from build123d import *

# Parameters (mm, degrees)
SKETCH2_R           = 11
SKETCH2_R_2         = 5
SKETCH2_R_3         = 1.5
SKETCH2_R_4         = 4
SKETCH2_R_5         = 1.75
SKETCH2_RX          = 4
SKETCH2_RY          = 4
SKETCH2_RX_2        = 1.5
SKETCH2_RY_2        = 1.499925
SKETCH2_RX_3        = 3.75
SKETCH2_RY_3        = 3.7498125
BOSS_EXTRUDE1_DEPTH = 2


with BuildPart() as part:
    # Sketch2 → Boss-Extrude1 (new body)
    with BuildSketch(Plane(origin=(0, 0, 0), x_dir=(1, 0, 0), z_dir=(0, 1, 0))):
        with BuildLine():
            Line((-106.00499968, 144.943614194), (182.962816245, 145.197156615))
            add(Edge.make_bspline(
                [(214.069631291, 100.332253712), (230.927799732, 145.239327045), (182.962816245, 145.197156615)],
                knots=[4.353250182, 4.353250182, 4.353250182, 6.284064455, 6.284064455, 6.284064455], degree=2, weights=[1, 0.569082143, 1]))
            Line((214.069631291, 100.332253712), (171.90071668, -12.000000001))
            add(Edge.make_bspline(
                [(160.992350179, -19), (168.692373591, -19.000128232), (171.90071668, -12.000000001)],
                knots=[3.141576001, 3.141576001, 3.141576001, 4.282613549, 4.282613549, 4.282613549], degree=2, weights=[1, 0.841620915, 1]))
            Line((160.992350179, -19), (-18.998606102, -18.99996049))
            add(Edge.make_bspline(
                [(-29.699861268, -12.428586042), (-26.366669696, -18.999958873), (-18.998606102, -18.99996049)],
                knots=[5.181825727, 5.181825727, 5.181825727, 6.283185508, 6.283185508, 6.283185508], degree=2, weights=[1, 0.852168955, 1]))
            Line((-29.699861268, -12.428586042), (-116.08526313, 126.611232779))
            add(Edge.make_bspline(
                [(-106.00499968, 144.943614194), (-127.678824036, 144.924558741), (-116.08526313, 126.611232779)],
                knots=[0.000879148, 0.000879148, 0.000879148, 2.135198153, 2.135198153, 2.135198153], degree=2, weights=[1, 0.482613975, 1]))
        make_face()
        with Locations((182.992000002, 111.999999999)):
            Circle(SKETCH2_R, mode=Mode.SUBTRACT)
        with Locations((-18.9988, 64)):
            Circle(SKETCH2_R_2, mode=Mode.SUBTRACT)
        with Locations((70.99645, 64)):
            Circle(SKETCH2_R_2, mode=Mode.SUBTRACT)
        with Locations((150.9927, 64)):
            Circle(SKETCH2_R_2, mode=Mode.SUBTRACT)
        with Locations((-78.996040132, 136.5)):
            Circle(SKETCH2_R_3, mode=Mode.SUBTRACT)
        with Locations((20.99895, 136.5)):
            Circle(SKETCH2_R_3, mode=Mode.SUBTRACT)
        with Locations((120.99395, 136.5)):
            Circle(SKETCH2_R_3, mode=Mode.SUBTRACT)
        with Locations((180.99095, 136.5)):
            Circle(SKETCH2_R_3, mode=Mode.SUBTRACT)
        with Locations((170.332531489, 6.118627774)):
            Circle(SKETCH2_R_3, mode=Mode.SUBTRACT)
        with Locations((177.330672341, 24.854456596)):
            Circle(SKETCH2_R_3, mode=Mode.SUBTRACT)
        with Locations((184.328557385, 43.589600555)):
            Circle(SKETCH2_R_3, mode=Mode.SUBTRACT)
        with Locations((191.32646769, 62.324812144)):
            Circle(SKETCH2_R_3, mode=Mode.SUBTRACT)
        with Locations((198.324441471, 81.060193672)):
            Circle(SKETCH2_R_3, mode=Mode.SUBTRACT)
        with Locations((-38.361920415, 16.671266638)):
            Circle(SKETCH2_R_3, mode=Mode.SUBTRACT)
        with Locations((-48.916261932, 33.658786529)):
            Circle(SKETCH2_R_3, mode=Mode.SUBTRACT)
        with Locations((-59.470762984, 50.646563195)):
            Circle(SKETCH2_R_3, mode=Mode.SUBTRACT)
        with Locations((-70.02547384, 67.634677545)):
            Circle(SKETCH2_R_3, mode=Mode.SUBTRACT)
        with Locations((-80.580283096, 84.622950275)):
            Circle(SKETCH2_R_3, mode=Mode.SUBTRACT)
        with Locations((70.99665, -7)):
            Circle(SKETCH2_R_4, mode=Mode.SUBTRACT)
        with Locations((120.99395, 0.5)):
            Circle(SKETCH2_R_5, mode=Mode.SUBTRACT)
        with Locations((20.99895, 0.5)):
            Circle(SKETCH2_R_5, mode=Mode.SUBTRACT)
        with Locations(Location((-105.9945, 133), (0, 0, 180))):
            Ellipse(SKETCH2_RX, SKETCH2_RY, mode=Mode.SUBTRACT)
        with Locations(Location((160.99255, -7), (0, 0, 90))):
            Ellipse(SKETCH2_RX, SKETCH2_RY, mode=Mode.SUBTRACT)
        with Locations(Location((182.99085, 126), (0, 0, 90))):
            Ellipse(SKETCH2_RX_2, SKETCH2_RY_2, mode=Mode.SUBTRACT)
        with Locations(Location((196.99015, 112), (0, 0, 90))):
            Ellipse(SKETCH2_RX_2, SKETCH2_RY_2, mode=Mode.SUBTRACT)
        with Locations(Location((168.99155, 112), (0, 0, 90))):
            Ellipse(SKETCH2_RX_2, SKETCH2_RY_2, mode=Mode.SUBTRACT)
        with Locations(Location((182.99085, 98), (0, 0, 90))):
            Ellipse(SKETCH2_RX_2, SKETCH2_RY_2, mode=Mode.SUBTRACT)
        with Locations(Location((120.99395, 64), (0, 0, 90))):
            Ellipse(SKETCH2_RX_2, SKETCH2_RY_2, mode=Mode.SUBTRACT)
        with Locations(Location((20.99895, 64), (0, 0, 90))):
            Ellipse(SKETCH2_RX_2, SKETCH2_RY_2, mode=Mode.SUBTRACT)
        with Locations(Location((-58.99705, 64), (0, 0, 90))):
            Ellipse(SKETCH2_RX_2, SKETCH2_RY_2, mode=Mode.SUBTRACT)
        with Locations(Location((180.99095, 64), (0, 0, 90))):
            Ellipse(SKETCH2_RX_2, SKETCH2_RY_2, mode=Mode.SUBTRACT)
        with Locations(Location((60.99695, 96.5), (0, 0, 90))):
            Ellipse(SKETCH2_RX_2, SKETCH2_RY_2, mode=Mode.SUBTRACT)
        with Locations(Location((140.99295, 96.5), (0, 0, 90))):
            Ellipse(SKETCH2_RX_2, SKETCH2_RY_2, mode=Mode.SUBTRACT)
        with Locations(Location((160.99195, 31.499978192), (0, 0, 90))):
            Ellipse(SKETCH2_RX_2, SKETCH2_RY_2, mode=Mode.SUBTRACT)
        with Locations(Location((80.99595, 31.499985778), (0, 0, 90))):
            Ellipse(SKETCH2_RX_2, SKETCH2_RY_2, mode=Mode.SUBTRACT)
        with Locations(Location((-18.99905, 96.5), (0, 0, 90))):
            Ellipse(SKETCH2_RX_2, SKETCH2_RY_2, mode=Mode.SUBTRACT)
        with Locations(Location((-38.99805, 31.499994311), (0, 0, 90))):
            Ellipse(SKETCH2_RX_2, SKETCH2_RY_2, mode=Mode.SUBTRACT)
        with Locations(Location((-101.689209002, 118.598380963), (0, 0, 90))):
            Ellipse(SKETCH2_RX_2, SKETCH2_RY_2, mode=Mode.SUBTRACT)
        with Locations(Location((-91.134705429, 101.610600241), (0, 0, 90))):
            Ellipse(SKETCH2_RX_2, SKETCH2_RY_2, mode=Mode.SUBTRACT)
        with Locations(Location((205.322481122, 99.795751553), (0, 0, 90))):
            Ellipse(SKETCH2_RX_2, SKETCH2_RY_2, mode=Mode.SUBTRACT)
        with Locations(Location((20.99895, 96.5), (0, 0, 90))):
            Ellipse(SKETCH2_RX_2, SKETCH2_RY_2, mode=Mode.SUBTRACT)
        with Locations(Location((100.99495, 96.5), (0, 0, 90))):
            Ellipse(SKETCH2_RX_2, SKETCH2_RY_2, mode=Mode.SUBTRACT)
        with Locations(Location((-58.99705, 96.5), (0, 0, 90))):
            Ellipse(SKETCH2_RX_2, SKETCH2_RY_2, mode=Mode.SUBTRACT)
        with Locations(Location((0.99995, 31.499992415), (0, 0, 90))):
            Ellipse(SKETCH2_RX_2, SKETCH2_RY_2, mode=Mode.SUBTRACT)
        with Locations(Location((40.99795, 31.499988622), (0, 0, 90))):
            Ellipse(SKETCH2_RX_2, SKETCH2_RY_2, mode=Mode.SUBTRACT)
        with Locations(Location((120.99395, 31.499981037), (0, 0, 90))):
            Ellipse(SKETCH2_RX_2, SKETCH2_RY_2, mode=Mode.SUBTRACT)
        with Locations(Location((-66.99665, 112), (0, 0, 90))):
            Ellipse(SKETCH2_RX_3, SKETCH2_RY_3, mode=Mode.SUBTRACT)
        with Locations(Location((57.9973, 112), (0, 0, 180))):
            Ellipse(SKETCH2_RX, SKETCH2_RY, mode=Mode.SUBTRACT)
        with Locations(Location((-5.9995, 133), (0, 0, 90))):
            Ellipse(SKETCH2_RX, SKETCH2_RY, mode=Mode.SUBTRACT)
        with Locations(Location((93.995420809, 133), (0, 0, 180))):
            Ellipse(SKETCH2_RX, SKETCH2_RY, mode=Mode.SUBTRACT)
        with BuildLine():
            Line((-18.998603467, -3), (1.00035, -3))
            add(Edge.make_bspline(
                [(1.00035, -11), (5.00035, -11), (5.00035, -7), (5.00035, -3), (1.00035, -3)],
                knots=[3.141592654, 3.141592654, 3.141592654, 4.71238898, 4.71238898, 6.283185307, 6.283185307, 6.283185307], degree=2, weights=[1, 0.707106781, 1, 0.707106781, 1]))
            Line((1.00035, -11), (-18.998603467, -11))
            add(Edge.make_bspline(
                [(-18.998603467, -3), (-22.998556935, -3), (-22.998556935, -7), (-22.998556935, -11), (-18.998603467, -11)],
                knots=[3.141592654, 3.141592654, 3.141592654, 4.71238898, 4.71238898, 6.283185307, 6.283185307, 6.283185307], degree=2, weights=[1, 0.707106781, 1, 0.707106781, 1]))
        make_face(mode=Mode.SUBTRACT)
    extrude(amount=BOSS_EXTRUDE1_DEPTH)


solid = part.part
Check sheet for the modelled part. Datum: model origin and axes. Units: mm. Round coordinates to 2 decimals unless told otherwise and drop trailing zeros. Loops run counter-clockwise (first coordinate to the right, second up) from the corner with the lowest first, then second, coordinate; pieces in that order, holes last. Notation, with made-up numbers: (3.25, 19.25) - (9.25, 19.25) arc R22 ccw to (9.25, 48.25) - close; hole circle Ø2 at (59.25, 69.25). An arc over 180 degrees is marked (long way). Answer as CSV lines item,"result". Start each with the question number.
Item 1: Section check C-C (x = -33). Record the boundary of the cut face in (y, z).
Item 2: Release check for a two-part mould opening along Z. For faces 1 (the flat face through (54, 0, -64)), 2 (the cylindrical face through (74.692, 0.986, 8.532)), 3 (the flat face through (-72.29, 0.99, -56.12)) record: +Z half, -Z half, draft (parallel to the pull), parting line (faces both ways), or undercut.
Item 3: Section check A-A (z = 7). Count the separate pieces of the cut face and the enclosed holes in it, and give its area (3 significant figures).
Item 4: Depth check by flat-ended pin: P1, Ø8, axis at x = 150.99, z = -64, coming from the +Y side; P2, Ø1, axis at x = -9, y = 1, coming from the -Z side. Enter the tip coordinate at first touch or a pass-through.
Item 5: Scan lines: line 1 (Z direction, x = 161, y = 1.35); line 2 (Z direction, x = -5.5, y = 0.4); line 3 (Z direction, x = 22, y = 1.95). Record each from-to range of solid material in increasing order. Write a range as [from, to].
Report:
1,outline,"(0, -145.01) - (2, -145.01) - (2, 7.12) - (0, 7.12) - close"
2,face 1,"draft"
2,face 2,"undercut"
2,face 3,"+Z half"
3,separate pieces,"4"
3,enclosed holes,"0"
3,area,"326 mm2"
4,P1,"passes through"
4,P2,"stops at z = -145.03"
5,line 1,"z = [-145.18, -33], [-30, 3], [11, 19]"
5,line 2,"z = [-145.03, -136.97], [-129.03, 3], [11, 19]"
5,line 3,"z = [-145.06, -137.62], [-135.38, -97.62], [-95.38, -65.12], [-62.88, -1.94], [0.94, 19]"
